Verification items for this drawing (mm, ordinates from the low corner). Coordinates: 2 decimals unless noted, no trailing zeros. Write each loop counter-clockwise with the first axis right and the second up, starting at its lowest first coordinate (ties: lowest second). Pieces come first, ordered by that corner, then holes. Notation, with made-up numbers: M -35,-21 L -14,-21 A15 cw -14,5 Z; hole C 88,-3 d11. An arc over 180 degrees is marked long. Put each result on its own line as item: value. Start each with the question number.
1) Gauge pin test, flat ends, axial feed: pin 1 (4 mm diameter, centred on x = 2, z = 10.5, fed in from -Y); pin 2 (2 mm diameter, centred on x = 3.5, y = 4, fed in from +Z). Record the tip position at first contact, or that the pin passes through.
2) Scan lines: line 1 along X through (y, z) = (4, 9.75); line 2 along Z through (x, y) = (4, 3.5); line 3 along Y through (x, z) = (3, 6.5). Record each from-to range of solid material in increasing order.
3) Mould release check, pull along Y, two halves, no side actions. Record for the marked faces 1, 2 and 3: released by +Y, released by -Y, zero draft, split by the parting line, or undercut.
4) Cross-section at D-D on y = 6.5. Record the cut outline in (x, z).
5) Cross-section at B-B on z = 10. Record the cut outline in (x, y).
6) Cross-section at C-C on x = 3.5. Record the cut outline in (y, z).
7) Cross-section at A-A on y = 4.75. Record the cut outline in (x, z).
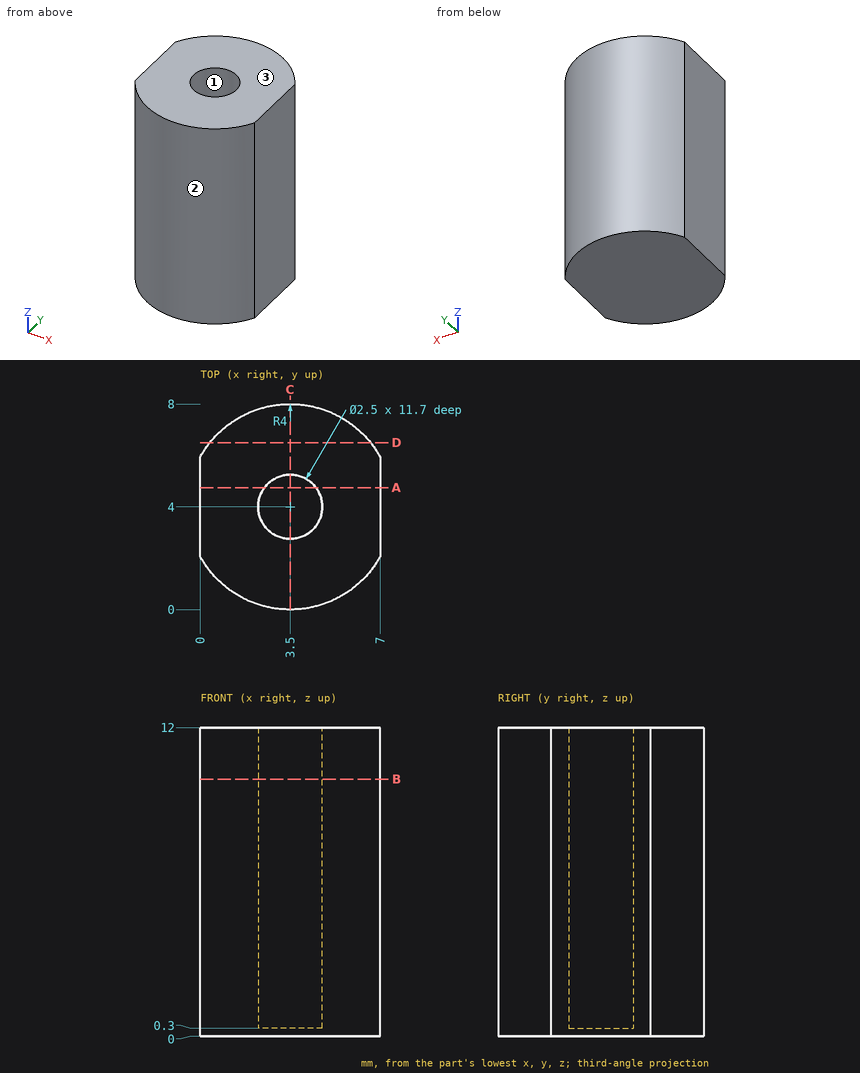
Answer key:
1. pin 1: stops at y = 0
1. pin 2: stops at z = 0.3
2. line 1: x = 0 to 2.25, 4.75 to 7
2. line 2: z = 0 to 0.3
2. line 3: y = 0.03 to 2.85, 5.15 to 7.97
3. face 1: undercut
3. face 2: released by -Y
3. face 3: zero draft
4. outline: M 0.38,0 L 6.62,0 L 6.62,12 L 0.38,12 Z
5. outline: M 0,2.06 A4 ccw 7,2.06 L 7,5.94 A4 ccw 0,5.94 Z; hole C 3.5,4 d2.5
6. outline: M 0,0 L 8,0 L 8,12 L 5.25,12 L 5.25,0.3 L 2.75,0.3 L 2.75,12 L 0,12 Z
7. outline: M 0,0 L 7,0 L 7,12 L 4.5,12 L 4.5,0.3 L 2.5,0.3 L 2.5,12 L 0,12 Z
